```python
from build123d import *

# Parameters (mm, degrees)
F1_ANGLE = 30
F2_COUNT = 4


with BuildPart() as f1:
    # F0 (on Front) → F1 (revolve)
    with BuildSketch(Plane.XZ):
        Polygon((7.366, 2.032), (7.366, 4.318), (8.382, 4.318), (7.366, 6.0777636205), (6.35, 6.0777636205), (6.35, 2.032), align=None)
    revolve(axis=Axis((0, 0, 1.016), (0, 0, -1)), revolution_arc=F1_ANGLE)


with BuildPart() as f2_1:
    # F2: instance of F1
    add(f1.part.rotate(Axis((0, 0, 1.016), (0, 0, -1)), 1 * 360 / F2_COUNT))


with BuildPart() as f2_2:
    # F2: instance of F1
    add(f1.part.rotate(Axis((0, 0, 1.016), (0, 0, -1)), 2 * 360 / F2_COUNT))


with BuildPart() as f2_3:
    # F2: instance of F1
    add(f1.part.rotate(Axis((0, 0, 1.016), (0, 0, -1)), 3 * 360 / F2_COUNT))


with BuildPart() as f1_1:
    add(f1.part)

    add(f2_1.part)  # F3 merges F2_1

    add(f2_2.part)  # F3 merges F2_2

    add(f2_3.part)  # F3 merges F2_3
    # F0 (on Front) → F3 (revolve)
    with BuildSketch(Plane.XZ):
        Polygon((8.382, 2.032), (7.366, 2.032), (6.35, 2.032), (0, 2.032), (0, 0), (8.382, 0), align=None)
    revolve(axis=Axis((0, 0, 1.016), (0, 0, -1)))


solid = f1_1.part
```
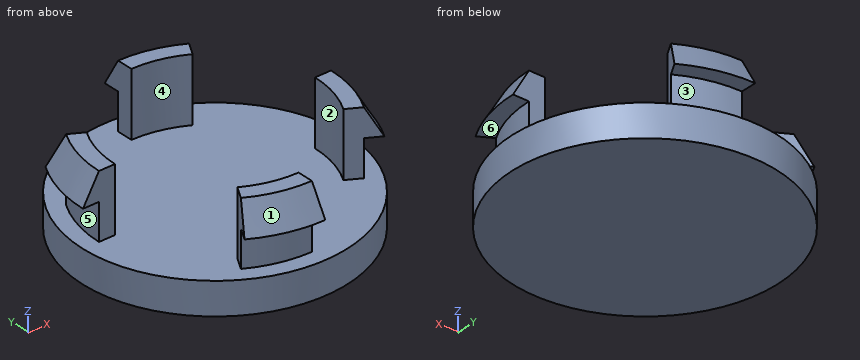
Source: CAD feature listing. Evaluate the final solid. Frame: model axes, mm. Face numbers are marked on the shaded views. A direction names the side the tool comes from. Round coordinates to 2 decimals unless told otherwise and drop trailing zeros. Loops run counter-clockwise (first coordinate to the right, second up) from the corner with the lowest first, then second, coordinate; pieces in that order, holes last. Notation, with made-up numbers: (3.25, -39) - (59.25, -39) arc R26 ccw to (59.25, -4) - close; hole circle Ø5 at (3.25, 69.5). An arc over 180 degrees is marked (long way). Use CSV: the item, a comma, the result in double quotes.
Q1. Mould query, pull axis Z, two halves, no side actions, for the marked faces 1, 2 and 3. Classes: pulls with the +Z half, pulls with the -Z half, needs draft (parallel to the pull), parting line crosses it, or undercut.
Reported:
face 1,"pulls with the +Z half"
face 2,"needs draft"
face 3,"undercut"
Q2. Ray query, line 1 along Z through (x, y) = (5, 4.5); line 2 along X through (y, z) = (4, 0.5); line 3 along Y through (x, z) = (-2.5, 2.5). Return the intervals inside material, ascending.
Reported:
line 1,"0 to 2.03"
line 2,"-7.37 to 7.37"
line 3,"-6.93 to -5.84"
Q3. Pin query (flat end, axial travel): pin 1 Ø2 at (y, z) = (-7, 4.5) entering from +X; pin 2 Ø1.5 at (x, z) = (6, 0.5) entering from +Y; pin 3 Ø1 at (y, z) = (-2, 2) entering from +X. Return the tip coordinate at first contact, or that it passes through.
Reported:
pin 1,"x = 0"
pin 2,"y = 6.53"
pin 3,"x = 8.25"
Q4. Section query B-B, the plane z = 1. Output: boundary loops of the cut face in (x, y).
Reported:
outline,"circle Ø16.76 at (0, 0)"
Q5. Reachability of the marked faces 4, 5 and 6 from +Z, -Z, +X, -X, +Y, -Y: full face, straight path, thin tool, end or side. Return the list, or none.
Reported:
face 4,"+Z, -X, -Y"
face 5,"-X, +Y"
face 6,"+X, -Y"
Q6. Section query A-A, the plane z = 4. Output: boundary loops of the cut face in (x, y) (3 decimals), then the cut area to 3 significant figures.
Reported:
outline,"(-7.366, 0) - (-6.35, 0) arc R6.35 cw to (-5.499, 3.175) - (-6.379, 3.683) arc R7.366 ccw to start; (-3.683, -6.379) arc R7.366 ccw to (0, -7.366) - (0, -6.35) arc R6.35 cw to (-3.175, -5.499) - close; (0, 6.35) arc R6.35 cw to (3.175, 5.499) - (3.683, 6.379) arc R7.366 ccw to (0, 7.366) - close; (5.499, -3.175) - (6.379, -3.683) arc R7.366 ccw to (7.366, 0) - (6.35, 0) arc R6.35 cw to start"
area,"14.6 mm^2"
Q7. Section query C-C, the plane y = -4.75. Output: boundary loops of the cut face in (x, z).
Reported:
outline,"(-6.91, 0) - (6.91, 0) - (6.91, 2.03) - (-6.91, 2.03) - close"
